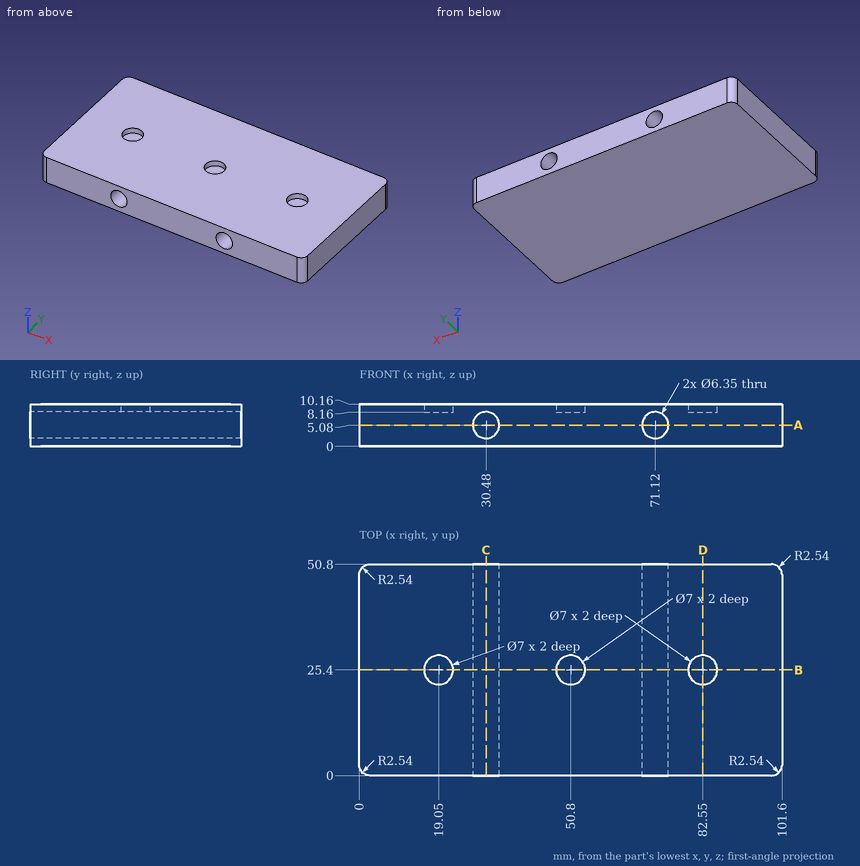
Check sheet for the drawn part. Datum: minimum x, y, z corner. Units: mm. Give positions to 0.01 mm unless a question says otherwise; leave off trailing zeros. Loops run counter-clockwise (first coordinate to the right, second up) from the corner with the lowest first, then second, coordinate; pieces in that order, holes last.
1) Sectioned sample at D-D, the plane x = 82.55. Enter the section's corners in (y, z), then the cut area to 3 significant figures.
2) Sectioned sample at B-B, the plane y = 25.4. Enter the section's corners in (x, z) (3 decimals).
3) Depth check by flat-ended pin: pin 1 Ø2 at (x, y) = (52, 25) entering from +Z. Enter the tip coordinate at first touch or a pass-through.
4) Sectioned sample at A-A, the plane z = 5.08. Enter the section's corners in (x, y) (3 decimals), then the cut area to 3 significant figures.
5) Sectioned sample at C-C, the plane x = 30.48. Enter the section's corners in (y, z) (3 decimals), then the cut area to 3 significant figures.
6) Thickness scan on line 1 along X through (y, z) = (25.4, 8.8); line 2 along X through (y, z) = (36, 3); line 3 along X through (y, z) = (37.5, 7.75). Record the ranges inside material, lowest first.
Answers:
1. outline: (0, 0) - (50.8, 0) - (50.8, 10.16) - (28.9, 10.16) - (28.9, 8.16) - (21.9, 8.16) - (21.9, 10.16) - (0, 10.16) - close
1. area: 502 mm2
2. outline: (0, 0) - (101.6, 0) - (101.6, 10.16) - (86.05, 10.16) - (86.05, 8.16) - (79.05, 8.16) - (79.05, 10.16) - (54.3, 10.16) - (54.3, 8.16) - (47.3, 8.16) - (47.3, 10.16) - (22.55, 10.16) - (22.55, 8.16) - (15.55, 8.16) - (15.55, 10.16) - (0, 10.16) - close; hole circle Ø6.35 at (30.48, 5.08); hole circle Ø6.35 at (71.12, 5.08)
3. pin 1: stops at z = 8.16
4. outline: (0, 2.54) arc R2.54 ccw to (2.54, 0) - (27.305, 0) - (27.305, 50.8) - (2.54, 50.8) arc R2.54 ccw to (0, 48.26) - close; (33.655, 0) - (67.945, 0) - (67.945, 50.8) - (33.655, 50.8) - close; (74.295, 0) - (99.06, 0) arc R2.54 ccw to (101.6, 2.54) - (101.6, 48.26) arc R2.54 ccw to (99.06, 50.8) - (74.295, 50.8) - close
4. area: 4,510 mm2
5. outline: (0, 0) - (50.8, 0) - (50.8, 1.905) - (0, 1.905) - close; (0, 8.255) - (50.8, 8.255) - (50.8, 10.16) - (0, 10.16) - close
5. area: 194 mm2
6. line 1: x = 0 to 15.55, 22.55 to 47.3, 54.3 to 79.05, 86.05 to 101.6
6. line 2: x = 0 to 28.08, 32.88 to 68.72, 73.52 to 101.6
6. line 3: x = 0 to 28.76, 32.2 to 69.4, 72.84 to 101.6
